The model under review builds one solid part; all positions refer to its coordinate system, in mm. Face numbers are marked on the shaded views. A direction names the side the tool comes from. Round coordinates to 2 decimals unless told otherwise and drop trailing zeros. Loops run counter-clockwise (first coordinate to the right, second up) from the corner with the lowest first, then second, coordinate; pieces in that order, holes last. Notation, with made-up numbers: (86, -31.5) - (95, -31.5) arc R19 cw to (95, -5.5) - close; hole circle Ø6 at (42, 50.5). An arc over 180 degrees is marked (long way). Answer as CSV lines item,"result".
from build123d import *
from OCP.BRepFilletAPI import BRepFilletAPI_MakeChamfer

# Parameters (mm, degrees)
SKETCH1_R           = 25
SKETCH1_R_2         = 14
SKETCH1_R_3         = 9.9
BOSS_EXTRUDE1_DEPTH = 3
SKETCH2_R           = 14
SKETCH2_R_2         = 9.9
BOSS_EXTRUDE2_DEPTH = 35
FILLET1_R           = 20
SKETCH3_R           = 2
CUT_EXTRUDE1_DEPTH  = 35
CUT_EXTRUDE2_START  = -4
SKETCH4_R           = 4
CUT_EXTRUDE2_DEPTH  = 18
CHAMFER1_SIZE       = 1
CHAMFER1_SIZE2      = 0.700207538
CUT_EXTRUDE3_REACH  = 53.904
SKETCH5_R           = 2
SKETCH5_R_2         = 4.790081367


with BuildPart() as part:
    # Sketch1 → Boss-Extrude1 (new body)
    # profile 1 of 2: a face of its own
    with BuildSketch(Plane.XY):
        Circle(SKETCH1_R)
        Circle(SKETCH1_R_2, mode=Mode.SUBTRACT)
    # profile 2 of 2: a face of its own
    with BuildSketch(Plane.XY):
        Circle(SKETCH1_R_2)
        Circle(SKETCH1_R_3, mode=Mode.SUBTRACT)
    extrude(amount=BOSS_EXTRUDE1_DEPTH)

    # Sketch2 → Boss-Extrude2 (add)
    with BuildSketch(Plane.XY.offset(3)):
        Circle(SKETCH2_R)
        Circle(SKETCH2_R_2, mode=Mode.SUBTRACT)
    extrude(amount=BOSS_EXTRUDE2_DEPTH)

    # Fillet1
    # the kernel refuses this fillet: 20 mm, written as the material it adds along each edge
    with BuildSketch(Plane(origin=(0, 0, 3), x_dir=(1, 0, 0), z_dir=(0, -1, 0))) as fillet1_piece_1:
        with BuildLine():
            CenterArc((34, 17.860571099), FILLET1_R, 180, 63.25631605)
            Line((14, 17.860571099), (13.6, 17.860571099))
            Line((13.6, 17.860571099), (13.6, 0))
            Line((13.6, 0), (14, -0.4))
            ThreePointArc((14, -0.4), (19.5, -0.4), (24.82, -0.357211422))
            Line((24.82, -0.357211422), (25, 0))
        make_face()
    revolve(axis=Axis((0, 0, 3), (0, 0, 1)))

    # Sketch3 → Cut-Extrude1 (cut)
    with BuildSketch(Plane(origin=(0, 0, 0), x_dir=(-1, 0, 0), z_dir=(0, 0, -1))):
        with Locations((0, 18.918658527)):
            Circle(SKETCH3_R)
        with Locations((16.38403889, -9.459329263)):
            Circle(SKETCH3_R)
        with Locations((-16.38403889, -9.459329263)):
            Circle(SKETCH3_R)
    extrude(amount=-CUT_EXTRUDE1_DEPTH, mode=Mode.SUBTRACT)

    # Sketch4 → Cut-Extrude2 (cut)
    with BuildSketch(Plane(origin=(0, 0, 0), x_dir=(-1, 0, 0), z_dir=(0, 0, -1)).offset(CUT_EXTRUDE2_START)):
        with Locations((-16.38403889, -9.459329263)):
            Circle(SKETCH4_R)
        with Locations((0, 18.918658527)):
            Circle(SKETCH4_R)
        with Locations((16.38403889, -9.459329263)):
            Circle(SKETCH4_R)
    extrude(amount=-CUT_EXTRUDE2_DEPTH, mode=Mode.SUBTRACT)

    # Chamfer1: one chamfer whose edges measure the first distance from different faces: ONE call of the kernel's chamfer builder (chamfer() names one face for all edges)
    chamfer1_edges_1 = [part.edges().sort_by_distance(p)[0] for p in [
        (18.38403889, -9.459329263, 4),
    ]]
    chamfer1_side_1 = [part.faces().sort_by_distance(p)[0] for p in [
        (20.270901805, -9.459329263, 4),
    ]]
    chamfer1_edges_2 = [part.edges().sort_by_distance(p)[0] for p in [
        (2, 18.918658527, 4),
    ]]
    chamfer1_side_2 = [part.faces().sort_by_distance(p)[0] for p in [
        (3.886862915, 18.918658527, 4),
    ]]
    chamfer1_edges_3 = [part.edges().sort_by_distance(p)[0] for p in [
        (-14.38403889, -9.459329263, 4),
    ]]
    chamfer1_side_3 = [part.faces().sort_by_distance(p)[0] for p in [
        (-12.497175975, -9.459329263, 4),
    ]]
    chamfer1 = BRepFilletAPI_MakeChamfer(part.part.solid().wrapped)
    for e in chamfer1_edges_1:
        chamfer1.Add(CHAMFER1_SIZE, CHAMFER1_SIZE2, e.wrapped, chamfer1_side_1[0].wrapped)  # the first distance lies on this face
    for e in chamfer1_edges_2:
        chamfer1.Add(CHAMFER1_SIZE, CHAMFER1_SIZE2, e.wrapped, chamfer1_side_2[0].wrapped)  # the first distance lies on this face
    for e in chamfer1_edges_3:
        chamfer1.Add(CHAMFER1_SIZE, CHAMFER1_SIZE2, e.wrapped, chamfer1_side_3[0].wrapped)  # the first distance lies on this face
    add(Compound.cast(chamfer1.Shape()), mode=Mode.REPLACE)

    # Sketch5 → Cut-Extrude3 (cut, up to next)
    with BuildSketch(Plane(origin=(0, 0, 0), x_dir=(1, 0, 0), z_dir=(0, 1, 0)), mode=Mode.PRIVATE) as cut_extrude3_sk1:
        with Locations(Location((-0.515660085, -30.731266932, 0), (0, 0, 270))):
            Circle(SKETCH5_R)
    cut_extrude3_tool1 = extrude(cut_extrude3_sk1.sketch, amount=-CUT_EXTRUDE3_REACH, mode=Mode.PRIVATE) & part.part
    # Sketch5 → Cut-Extrude3 (cut, up to next)
    with BuildSketch(Plane(origin=(0, 0, 0), x_dir=(1, 0, 0), z_dir=(0, 1, 0)), mode=Mode.PRIVATE) as cut_extrude3_sk2:
        Circle(SKETCH5_R_2)
    cut_extrude3_tool2 = extrude(cut_extrude3_sk2.sketch, amount=-CUT_EXTRUDE3_REACH, mode=Mode.PRIVATE) & part.part
    add(cut_extrude3_tool1.solids().sort_by_distance((-0.51566, 0, 30.731267))[0], mode=Mode.SUBTRACT)
    add(cut_extrude3_tool2.solids().sort_by_distance((0, 0, 0))[0], mode=Mode.SUBTRACT)


solid = part.part
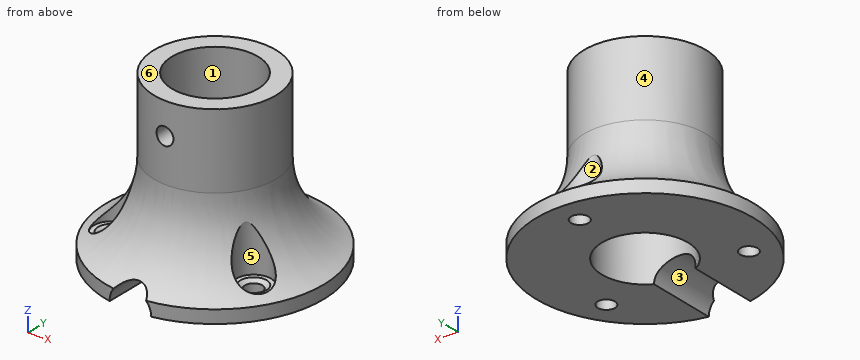
1. Draft analysis for pull direction Y (two halves, no side actions). For the marked faces 1, 2, 3 and 4, state which applies: +Y half, -Y half, draft (parallel to the pull), parting line (faces both ways), or undercut.
Numbers:
face 1,"undercut"
face 2,"undercut"
face 3,"draft"
face 4,"parting line"
2. Tool access review of the marked faces 5 and 6: name each direction out of +Z, -Z, +X, -X, +Y, -Y from which nothing blocks a thin tool from reaching the whole face with its end or side.
Numbers:
face 5,"+Z"
face 6,"+Z, +X, -X, +Y, -Y"
3. Clearance check with flat-ended pins moving along their axes: pin 1 (10.5 mm diameter, centred on x = 0, y = 18.92, fed in from +Z); pin 2 (4 mm diameter, centred on x = -1, y = 19.5, fed in from +Z); pin 3 (6 mm diameter, centred on x = -16.5, z = 5, fed in from +Y); pin 4 (12 mm diameter, centred on y = -8.5, z = 32.5, fed in from -X) (3 decimals). State where each tip first meets the part, or that it passes through.
Numbers:
pin 1,"stops at z = 38"
pin 2,"stops at z = 4"
pin 3,"stops at y = 20.53"
pin 4,"stops at x = -13.775"
4. Take a section at A-A (y = 0). State the section outline as (x, z) points, plus the area to 3 significant figures.
Numbers:
outline,"(-25, 0) - (-9.9, 0) - (-9.9, 38) - (-14, 38) - (-14, 20.86) arc R20 cw to (-25, 3) - close; (9.9, 0) - (25, 0) - (25, 3) arc R20 cw to (14, 20.86) - (14, 38) - (9.9, 38) - close"
area,"490 mm²"
5. Take a section at D-D (z = 17.5). State the section outline as (x, y) points, plus the area to 3 significant figures.
Numbers:
outline,"circle Ø28.57 at (0, 0); hole circle Ø19.8 at (0, 0)"
area,"333 mm²"
6. Take a section at B-B (z = 10). State the section outline as (x, y) points.
Numbers:
outline,"(-16.32, -5.46) arc R4 cw to (-12.89, -11.4) arc R17.21 ccw to (12.89, -11.4) arc R4 cw to (16.32, -5.46) arc R17.21 ccw to (3.43, 16.86) arc R4 cw to (-3.43, 16.86) arc R17.21 ccw to start; hole circle Ø19.8 at (0, 0)"
7. Wall thickness on probe 1 along X at (y, z) = (0.5, 2) (3 decimals); probe 2 along Y at (x, z) = (0, 2); probe 3 along X at (y, z) = (9, 17): over which ranges is each line inside the solid? List them lowest first.
Numbers:
probe 1,"x = -24.995 to -9.887, 9.887 to 24.995"
probe 2,"y = 9.9 to 16.92, 20.92 to 25"
probe 3,"x = -11.21 to -4.12, 4.12 to 11.21"
8. Take a section at C-C (z = 25.5). State the section outline as (x, y) points.
Numbers:
outline,"circle Ø28 at (0, 0); hole circle Ø19.8 at (0, 0)"
